Check sheet for the modelled part. Datum: model origin and axes. Units: mm. A direction names the side the tool comes from. Give positions to 0.01 mm unless a question says otherwise; leave off trailing zeros. Write each loop counter-clockwise with the first axis right and the second up, starting at its lowest first coordinate (ties: lowest second). Pieces come first, ordered by that corner, then holes. Notation, with made-up numbers: (66.25, 76.25) -> (124.25, 76.25) arc R34 ccw to (124.25, 110.25) -> close; hole circle Ø2 at (60.25, -35). An arc over 180 degrees is marked (long way). Use a Markdown table: item, result. Add a question column.
1. Set-up check for faces 1 (the flat face through (1.833, -11.238, 5.497)), 2 (the flat face through (0, 0.5, -14)), 3 (the flat face through (-8.63, 7.43, 5.5)), 4 (the flat face through (5.13, 2.2, 5.91)), 5 (the cylindrical face through (-8, -6, 5)): record each of +Z, -Z, +X, -X, +Y, -Y from which the full face is reachable in a straight line by a thin tool's end or side.
2. Gauge pin test, flat ends, axial feed: P1, Ø6, axis at x = -5, z = 5.5, coming from the -Y side; P2, Ø0.9, axis at x = -0.5, z = -13, coming from the -Y side; P3, Ø2.5, axis at x = 1, z = -13.5, coming from the +Y side. Record the tip position at first contact, or that the pin passes through.
3. Release check for a two-part mould opening along X. For faces 6 (the flat face through (-4.13, 10.61, 5.5)), 7 (the flat face through (-12.774, 1.352, 5.497)), 8 (the flat face through (8.834, -7.24, 5.497)) record: released by +X, released by -X, zero draft, split by the parting line, or undercut.
4. Cross-section at C-C (y = 5). Enter the section's corners in (x, z).
5. Scan lines: probe 1 along Y at (x, z) = (-10.25, 5); probe 2 along Z at (x, y) = (-8, -1); probe 3 along Z at (x, y) = (7.25, -2.25). Record each from-to range of solid material in increasing order. Write a range as [from, to].
6. Cross-section at B-B (y = 0). Enter the section's corners in (x, z).
7. Cross-section at A-A (z = -5.5). Enter the section's corners in (x, y).
from build123d import *

# Parameters (mm, degrees)
ESQUISSE1_R                        = 10
MAIN_EXTRUSION_DEPTH               = 10.841776527
GEAR_ELEMENT_DEPTH                 = 10.841776527
CONG_1_R                           = 0.3
R_P_TITION_CIRCULAIRE1_COUNT       = 9
R_P_TITION_CIRCULAIRE1_ANGLE       = 224
CONG_1_OF_R_P_TITION_CIRCULAIRE1_R = 0.3
ESQUISSE3_R                        = 4
MAIN_AXE_DEPTH                     = 15
ESQUISSE4_W                        = 5
ESQUISSE4_H                        = 1
AXE_TRAIT_DEPTH                    = 3
ENL_V_MAT_EXTRU_1_DEPTH            = 10


with BuildPart() as part:
    # Esquisse1 → Main Extrusion (new body)
    with BuildSketch(Plane.XY):
        Circle(ESQUISSE1_R)
    extrude(amount=MAIN_EXTRUSION_DEPTH)

    # Esquisse2 → Gear Element (add)
    with BuildSketch(Plane.XY.offset(10.841776527)):
        Polygon((-1.75, 9.845684334), (1.75, 9.845684334), (0.9, 12.845684334), (-0.9, 12.845684334), align=None)
    gear_element = extrude(amount=-GEAR_ELEMENT_DEPTH)

    # Congé1
    cong_1_edges = [part.edges().sort_by_distance(p)[0] for p in [
        (-1.75, 9.845684334, 5.420888263),
        (-0.9, 12.845684334, 5.420888263),
        (0.9, 12.845684334, 5.420888263),
        (1.75, 9.845684334, 5.420888263),
    ]]
    fillet(cong_1_edges, radius=CONG_1_R)

    # Répétition circulaire1: Gear Element ×9 about axis
    r_p_tition_circulaire1_axis = Axis((0, 0, 0), (0, 0, 1))
    for i in range(1, R_P_TITION_CIRCULAIRE1_COUNT):
        add(gear_element.rotate(r_p_tition_circulaire1_axis, i * R_P_TITION_CIRCULAIRE1_ANGLE / (R_P_TITION_CIRCULAIRE1_COUNT - 1)))

    # Congé1 of Répétition circulaire1
    cong_1_of_r_p_tition_circulaire1_edges = [part.edges().sort_by_distance(p)[0] for p in [
        (-6.167427098, 7.871648048, 5.420888263),
        (-6.825336333, 10.919541655, 5.420888263),
        (-5.236030666, 11.764590468, 5.420888263),
        (-3.077110523, 9.514798517, 5.420888263),
        (-9.141029821, 4.054821057, 5.420888263),
        (-11.152828571, 6.437081704, 5.420888263),
        (-10.146281345, 7.929349335, 5.420888263),
        (-7.183854659, 6.956452561, 5.420888263),
        (-9.974673456, -0.711259064, 5.420888263),
        (-12.869389948, 0.447669937, 5.420888263),
        (-12.681238714, 2.237809349, 5.420888263),
        (-9.608823834, 2.76956757, 5.420888263),
        (-8.473198013, -5.310830014, 5.420888263),
        (-11.573165181, -5.646543517, 5.420888263),
        (-12.247457049, -3.977612579, 5.420888263),
        (-9.78432109, -2.065686523, 5.420888263),
        (-4.988106123, -8.66711009, 5.420888263),
        (-7.567606729, -10.418873951, 5.420888263),
        (-8.946486726, -9.261856253, 5.420888263),
        (-7.669261674, -6.417353456, 5.420888263),
        (-0.335274576, -9.994377968, 5.420888263),
        (-1.790435109, -12.752095833, 5.420888263),
        (-3.55110079, -12.377854789, 5.420888263),
        (-3.758791178, -9.26668705, 5.420888263),
        (4.396046364, -8.981913848, 5.420888263),
        (4.40588599, -12.099990688, 5.420888263),
        (2.675614937, -12.596137928, 5.420888263),
        (1.031630428, -9.946644593, 5.420888263),
        (8.098231686, -5.866740455, 5.420888263),
        (9.570767967, -8.61521947, 5.420888263),
        (8.275956326, -9.865604537, 5.420888263),
        (5.580542385, -8.298044751, 5.420888263),
    ]]
    fillet(cong_1_of_r_p_tition_circulaire1_edges, radius=CONG_1_OF_R_P_TITION_CIRCULAIRE1_R)

    # Esquisse3 → Main Axe (add)
    with BuildSketch(Plane(origin=(0, 0, 0), x_dir=(-1, 0, 0), z_dir=(0, 0, -1))):
        with Locations(Location((0, 0, 0), (0, 0, 180))):
            Circle(ESQUISSE3_R)
    extrude(amount=MAIN_AXE_DEPTH)

    # Esquisse4 → Axe Trait (cut)
    with BuildSketch(Plane(origin=(0, 0, -15), x_dir=(-1, 0, 0), z_dir=(0, 0, -1))):
        Rectangle(ESQUISSE4_W, ESQUISSE4_H)
    extrude(amount=-AXE_TRAIT_DEPTH, mode=Mode.SUBTRACT)

    # Esquisse5 → Enlèv. mat.-Extru.1 (cut)
    with BuildSketch(Plane.XY.offset(10.841776527)):
        Polygon((0.854113079, 12.78498982), (9.495597726, -8.603435225), (13.592580869, -6.948146588), (4.951096222, 14.440278457), align=None)
    extrude(amount=-ENL_V_MAT_EXTRU_1_DEPTH, mode=Mode.SUBTRACT)


solid = part.part
Worked answers:
| question | item | result |
|---|---|---|
| 1 | face 1 | +Z, -Z, -Y |
| 1 | face 2 | -Z |
| 1 | face 3 | +Z, -Z, +Y |
| 1 | face 4 | +Z, +X, +Y |
| 1 | face 5 | +Z, -Z |
| 2 | P1 | stops at y = -12.71 |
| 2 | P2 | stops at y = -4 |
| 2 | P3 | stops at y = 4 |
| 3 | face 6 | undercut |
| 3 | face 7 | released by -X |
| 3 | face 8 | released by +X |
| 4 | outline | (-9.94, 0) -> (8.66, 0) -> (8.66, 0.84) -> (4, 0.84) -> (4, 10.84) -> (-9.94, 10.84) -> close |
| 5 | probe 1 | y = [-5.5, -2.43], [-0.6, 2.66], [5.37, 7.77] |
| 5 | probe 2 | z = [0, 10.84] |
| 5 | probe 3 | z = [0, 0.84] |
| 6 | outline | (-11.75, 0) -> (-4, 0) -> (-4, -15) -> (-2.5, -15) -> (-2.5, -12) -> (2.5, -12) -> (2.5, -15) -> (4, -15) -> (4, 0) -> (10, 0) -> (10, 0.84) -> (6.02, 0.84) -> (6.02, 10.84) -> (-11.75, 10.84) -> close |
| 7 | outline | circle Ø8 at (0, 0) |
